Build history of the part. All positions in model axes, mm. A direction names the side the tool comes from. Round coordinates to 2 decimals unless told otherwise and drop trailing zeros. Loops run counter-clockwise (first coordinate to the right, second up) from the corner with the lowest first, then second, coordinate; pieces in that order, holes last.
Autodesk Inventor part; units mm, degrees
ref_plane "YZ Plane" through (0, 0, 0) normal (1, 0, 0) x (0, 1, 0)
ref_plane "XZ Plane" through (0, 0, 0) normal (0, 1, 0) x (-1, 0, 0)
ref_plane "XY Plane" through (0, 0, 0) normal (0, 0, 1) x (1, 0, 0)
sketch "Sketch1" plane through (0, 0, 0) normal (0, 1, 0) x (-1, 0, 0)
  line L0 (6.35, 0) -> (44.45, 0)
  line L1 (50.8, -6.35) -> (50.8, -38.1)
  line L2 (50.8, -38.1) -> (0, -38.1)
  line L3 (0, -38.1) -> (0, -6.35)
  arc A0 (50.8, -6.35) -> (44.45, 0) centre (44.45, -6.35) ccw
  arc A1 (6.35, 0) -> (0, -6.35) centre (6.35, -6.35) ccw
  point P0 (0, 0)
  point P1 (50.8, 0)
  dimension "d0" = 50.8
  dimension "d1" = 38.1
  dimension "d2" = 6.35
  dimension "d3" = 6.35
extrude "Extrusion1" add sketch "Sketch1" along normal blind 12.7
sketch "Sketch2" plane through (0, 0, -38.1) normal (0, 0, -1) x (-1, 0, 0)
  circle A0 centre (25.4, 57.15) radius 6.35
  circle A1 centre (25.4, 57.15) radius 12.7
  line L0 (38.1, 25.4) -> (38.1, 57.15)
  line L1 (12.7, 57.15) -> (12.7, 25.4)
  line L2 (0, 12.7) -> (50.8, 12.7)
  line L3 (6.35, 12.7) -> (0, 12.7)
  arc A2 (0, 12.7) -> (12.7, 25.4) centre (0, 25.4) ccw
  arc A3 (38.1, 25.4) -> (50.8, 12.7) centre (50.8, 25.4) ccw
  point P0 (0, 0)
  point P1 (25.4, 12.7)
  dimension "d6" = 12.7
  dimension "d7" = 25.4
  dimension "d12" = 44.45
extrude "Extrusion2" add sketch "Sketch2" against normal blind 12.7 contours L0 A3 L2 A2 L1 A1
extrude "Extrusion3" add sketch "Sketch2" against normal blind 25.4 contours A1
sketch "Sketch3" plane through (0, 12.7, 0) normal (0, 1, 0) x (1, 0, 0)
  circle A0 centre (-38.1, 12.7) radius 6.35
  circle A1 centre (-12.7, 12.7) radius 6.35
  line L0 (-44.45, 0) -> (-6.35, 0)
  line L1 (0, 6.35) -> (0, 25.4)
  line L2 (-50.8, 25.4) -> (-50.8, 6.35)
  point P0 (0, 0)
  dimension "d17" = 12.7
  dimension "d18" = 12.7
  dimension "d19" = 12.7
  dimension "d20" = 12.7
  dimension "d21" = 12.7
  dimension "d22" = 12.7
extrude "Extrusion4" cut sketch "Sketch3" against normal through all
properties part number "7.1 Part 5"
(1) Probe line 1 (X direction, y = 6, z = -12.7); line 2 (Z direction, x = -12.7, y = 4.5); line 3 (Y direction, x = -31, z = -24). List the from-to ranges inside material, lowest first.
Responses:
line 1: x = -50.8 to -44.45, -31.75 to -19.05, -6.35 to 0
line 2: z = -38.1 to -19.05, -6.35 to 0
line 3: y = 0 to 12.7, 45.75 to 54.16, 60.14 to 68.55
(2) Slice it at A-A on x = -25.4. List the corners of the cut face in (y, z), plus the area to 3 significant figures.
Responses:
outline: (0, -38.1) - (50.8, -38.1) - (50.8, -12.7) - (44.45, -12.7) - (44.45, -25.4) - (12.7, -25.4) - (12.7, 0) - (0, 0) - close; (63.5, -38.1) - (69.85, -38.1) - (69.85, -12.7) - (63.5, -12.7) - close
area: 1,210 mm2
(3) Slice it at C-C on y = 55. List the corners of the cut face in (x, z).
Responses:
outline: (-38.1, -38.1) - (-31.37, -38.1) - (-31.37, -12.7) - (-37.92, -12.7) - (-37.92, -25.4) - (-38.1, -25.4) - close; (-19.43, -38.1) - (-12.7, -38.1) - (-12.7, -25.4) - (-12.88, -25.4) - (-12.88, -12.7) - (-19.43, -12.7) - close
(4) Slice it at D-D on z = -24. List the corners of the cut face in (x, y).
Responses:
outline: (-50.8, 0) - (0, 0) - (0, 12.7) - (-50.8, 12.7) - close; circle Ø25.4 at (-25.4, 57.15); hole circle Ø12.7 at (-25.4, 57.15)
(5) Slice it at B-B on z = -16. List the corners of the cut face in (x, y), plus the area to 3 significant figures.
Responses:
outline: (-50.8, 0) - (-43.53, 0) - (-43.53, 12.7) - (-50.8, 12.7) - close; circle Ø25.4 at (-25.4, 57.15); (-32.67, 0) - (-18.13, 0) - (-18.13, 12.7) - (-32.67, 12.7) - close; (-7.27, 0) - (0, 0) - (0, 12.7) - (-7.27, 12.7) - close; hole circle Ø12.7 at (-25.4, 57.15)
area: 750 mm2
(6) Which spindle directions (+Z, -Z, +X, -X, +Y, -Y) get a long thin tool onto all of the face, cutting with end or side? Do faces 4 (the face through (-25, 12.7, -13)), 5 (the face through (-9.286, 6.439, -18.054)), 6 (the face through (-23.747, 69.742, -22.756)), 7 (the face through (-22, 63, -12.7)). Say none if no direction does.
Responses:
face 4: +Z, +X, -X
face 5: -Y
face 6: +Z
face 7: +Z, +X, -X, +Y
(7) Pull direction X, two halves, no side cores. Call faces 1 (the face through (-12.7, 41, -32)), 2 (the face through (-38.1, 41, -32)), 3 (the face through (-34.686, 6.439, -18.054)): +X half, -X half, draft (parallel to the pull), parting line (faces both ways), or undercut.
Responses:
face 1: +X half
face 2: -X half
face 3: undercut
(8) Pin check, flat tips, straight feed: P1, Ø8, axis at x = -36, y = 30, coming from the +Z side; P2, Ø14, axis at y = 37.5, z = -29.5, coming from the +X side; P3, Ø5, axis at y = 20.5, z = -29.5, coming from the -X side; P4, Ø14.5, axis at x = -38.1, z = -12.7, coming from the -Y side. Stop position of each tip, or through.
Responses:
P1: stops at z = -25.4
P2: stops at x = -12.7
P3: stops at x = -40.48
P4: stops at y = 0
